```python
from build123d import *

# Parameters (mm, degrees)
SKETCH1_W           = 45
SKETCH1_H           = 17
BOSS_EXTRUDE1_DEPTH = 2.5
SKETCH2_W           = 45
SKETCH2_H           = 17
SKETCH2_W_2         = 40
SKETCH2_H_2         = 12
BOSS_EXTRUDE2_DEPTH = 4.5
SKETCH3_R           = 0.957368162
SKETCH3_R_2         = 1.102212996
CUT_EXTRUDE1_DEPTH  = 46
SKETCH4_W           = 2.5
SKETCH4_H           = 17
BOSS_EXTRUDE3_DEPTH = 3
BOSS_EXTRUDE4_START = -2.5
BOSS_EXTRUDE4_DEPTH = 2.5
BOSS_EXTRUDE5_DEPTH = 2.5
SKETCH7_R           = 2.5
CUT_EXTRUDE2_DEPTH  = 2.5


with BuildPart() as part:
    # Sketch1 → Boss-Extrude1 (new body)
    with BuildSketch(Plane(origin=(0, 0, 0), x_dir=(1, 0, 0), z_dir=(0, 1, 0))):
        Rectangle(SKETCH1_W, SKETCH1_H)
    extrude(amount=BOSS_EXTRUDE1_DEPTH)

    # Sketch2 → Boss-Extrude2 (add)
    with BuildSketch(Plane.XZ):
        Rectangle(SKETCH2_W, SKETCH2_H)
        Rectangle(SKETCH2_W_2, SKETCH2_H_2, mode=Mode.SUBTRACT)
    extrude(amount=BOSS_EXTRUDE2_DEPTH)

    # Sketch3 → Cut-Extrude1 (cut, through all)
    with BuildSketch(Plane(origin=(22.5, 0, 0), x_dir=(0, 0, -1), z_dir=(1, 0, 0))):
        with Locations((-3.5, -2.5)):
            Circle(SKETCH3_R)
        with Locations((3.5, -2.5)):
            Circle(SKETCH3_R_2)
    extrude(amount=-CUT_EXTRUDE1_DEPTH, mode=Mode.SUBTRACT)

    # Sketch4 → Boss-Extrude3 (add)
    with BuildSketch(Plane.XZ.offset(4.5)):
        with Locations((-21.25, 0)):
            Rectangle(SKETCH4_W, SKETCH4_H)
        with Locations((21.25, 0)):
            Rectangle(SKETCH4_W, SKETCH4_H)
    extrude(amount=BOSS_EXTRUDE3_DEPTH)

    # Sketch5 → Boss-Extrude4 (add)
    with BuildSketch(Plane.XY.offset(8.5).offset(BOSS_EXTRUDE4_START)):
        Polygon((20, -7.5), (20, -4.5), (17, -4.5), align=None)
        Polygon((-20, -7.5), (-20, -4.5), (-17.287649909, -4.5), align=None)
    extrude(amount=BOSS_EXTRUDE4_DEPTH)

    # Sketch6 → Boss-Extrude5 (add)
    with BuildSketch(Plane(origin=(0, 0, -8.5), x_dir=(-1, 0, 0), z_dir=(0, 0, -1))):
        Polygon((20, -4.5), (17.287649909, -4.5), (20, -7.5), align=None)
        Polygon((-17, -4.5), (-20, -4.5), (-20, -7.5), align=None)
    extrude(amount=-BOSS_EXTRUDE5_DEPTH)

    # Sketch7 → Cut-Extrude2 (cut)
    with BuildSketch(Plane(origin=(0, 2.5, 0), x_dir=(1, 0, 0), z_dir=(0, 1, 0))):
        with Locations((-12.5, 0)):
            Circle(SKETCH7_R)
        with Locations((12.5, 0)):
            Circle(SKETCH7_R)
    cut_extrude2 = extrude(amount=-CUT_EXTRUDE2_DEPTH, mode=Mode.SUBTRACT)

    # Mirror1: Cut-Extrude2 across plane
    add(cut_extrude2.mirror(Plane.XY), mode=Mode.SUBTRACT)


solid = part.part
```
Here's how the part is built. I have some questions about the finished solid (model axes, mm). A direction names the side the tool comes from. Coordinates: 2 decimals unless noted, no trailing zeros. Order: outer loops, then holes, each group sorted by start corner. A loop starts at its lowest first (then second) coordinate and runs counter-clockwise, first axis right, second up.
1) Imagine slicing it at A-A on y = -2.5. List the corners of the cut face in (x, z) for me, and give its area (3 significant figures).
2) Imagine slicing it at C-C on x = 12.5. List the corners of the cut face in (y, z) for me, and give its area (3 significant figures).
3) Will these pins go through, and if not, where does the flat tip stop? pin 1 (6 mm diameter, centred on x = -4.5, z = 0, fed in from -Y); pin 2 (3 mm diameter, centred on x = 7.5, z = -8, fed in from -Y); pin 3 (3 mm diameter, centred on x = -12, z = -1, fed in from +Y).
4) Imagine slicing it at B-B on z = -3.5. List the corners of the cut face in (x, y) for me, and give its area (3 significant figures).
5) Which directions (+Z, -Z, +X, -X, +Y, -Y) give clear straight access to the entire face, cutting with the end or side of a thin tool? Please do faces 1 (the face through (-18.625, -5.979, -7.268)), 2 (the face through (-21.23, -2.92, -4.52)), 3 (the face through (20, -4, 0)).
6) I need wall thicknesses on line 1 (Y direction, x = -20.9, z = 3.5); line 2 (X direction, y = -5.5, z = -2.5); line 3 (Z direction, x = -12.5, y = 1.55). Which ranges of each line are inside material? Lowest first, please.
7) Imagine slicing it at D-D on y = 0.5. List the corners of the cut face in (x, z) for me, and give its area (3 significant figures).
8) We'd pull the mould along X, two halves only. Please class faces 4 (the face through (-18.625, -5.979, 7.232)), 5 (the face through (22.5, -2, 0)), 6 (the face through (-21.232, -3.435, 3.708)): +X half, -X half, draft (parallel to the pull), parting line (faces both ways), or undercut.
Response values:
1. outline: (-22.5, -8.5) - (22.5, -8.5) - (22.5, -4.6) - (20, -4.6) - (20, -6) - (-20, -6) - (-20, -4.6) - (-22.5, -4.6) - close; (-22.5, -2.4) - (-20, -2.4) - (-20, 2.54) - (-22.5, 2.54) - close; (-22.5, 4.46) - (-20, 4.46) - (-20, 6) - (20, 6) - (20, 4.46) - (22.5, 4.46) - (22.5, 8.5) - (-22.5, 8.5) - close; (20, -2.4) - (22.5, -2.4) - (22.5, 2.54) - (20, 2.54) - close
1. area: 264 mm2
2. outline: (-4.5, -8.5) - (2.5, -8.5) - (2.5, -2.5) - (0, -2.5) - (0, -6) - (-4.5, -6) - close; (-4.5, 6) - (0, 6) - (0, 2.5) - (2.5, 2.5) - (2.5, 8.5) - (-4.5, 8.5) - close
2. area: 52.5 mm2
3. pin 1: stops at y = 0
3. pin 2: stops at y = -4.5
3. pin 3: stops at y = 2.5
4. outline: (-22.5, -7.5) - (-20, -7.5) - (-20, -3.6) - (-22.5, -3.6) - close; (-22.5, -1.4) - (-20, -1.4) - (-20, 0) - (20, 0) - (20, -1.4) - (22.5, -1.4) - (22.5, 2.5) - (-22.5, 2.5) - close; (20, -7.5) - (22.5, -7.5) - (22.5, -3.6) - (20, -3.6) - close
4. area: 139 mm2
5. face 1: +Z, -Z, -Y
5. face 2: +X, -X
5. face 3: -Y
6. line 1: y = -7.5 to -3.46, -1.54 to 2.5
6. line 2: x = -22.5 to -20, 20 to 22.5
6. line 3: z = -8.5 to -2.5, 2.5 to 8.5
7. outline: (-22.5, -8.5) - (22.5, -8.5) - (22.5, 8.5) - (-22.5, 8.5) - close; hole circle Ø5 at (-12.5, 0); hole circle Ø5 at (12.5, 0)
7. area: 726 mm2
8. face 4: undercut
8. face 5: +X half
8. face 6: draft
